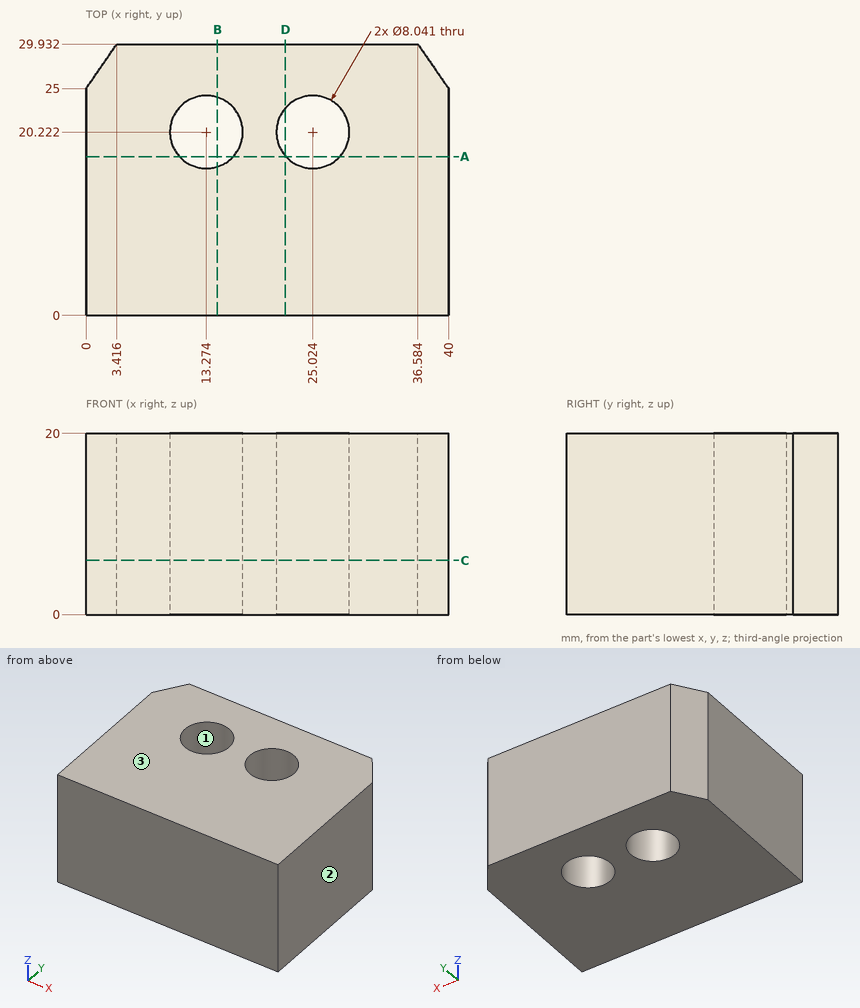
Study the drawing (mm; zero at the part's minimum x, y, z) and answer. Coordinates: 2 decimals unless noted, no trailing zeros. Write each loop counter-clockwise with the first axis right and the second up, starting at its lowest first coordinate (ties: lowest second). Pieces come first, ordered by that corner, then holes.
Q1. The mould has two halves that part along X. Classify the marked faces 1, 2 and 3: released by +X, released by -X, zero draft, split by the parting line, or undercut.
Returned:
face 1: undercut
face 2: released by +X
face 3: zero draft
Q2. Section B-B, the plane x = 14.5 is taken. Write down the section's boundary in (y, z).
Returned:
outline: (0, 0) - (16.39, 0) - (16.39, 20) - (0, 20) - close; (24.05, 0) - (29.93, 0) - (29.93, 20) - (24.05, 20) - close
Q3. Find the intervals of material crossed by line 1 along X through (y, z) = (22, 16.25); line 2 along X through (y, z) = (21, 2.25); line 3 along Y through (x, z) = (25, 11.5), in increasing order.
Returned:
line 1: x = 0 to 9.67, 16.88 to 21.42, 28.63 to 40
line 2: x = 0 to 9.33, 17.22 to 21.08, 28.97 to 40
line 3: y = 0 to 16.2, 24.24 to 29.93
Q4. Section C-C, the plane z = 6 is taken. Write down the section's boundary in (x, y) (1 decimal).
Returned:
outline: (0, 0) - (40, 0) - (40, 25) - (36.6, 29.9) - (3.4, 29.9) - (0, 25) - close; hole circle Ø8 at (13.3, 20.2); hole circle Ø8 at (25, 20.2)
Q5. Section D-D, the plane x = 22 is taken. Write down the section's boundary in (y, z).
Returned:
outline: (0, 0) - (17.57, 0) - (17.57, 20) - (0, 20) - close; (22.87, 0) - (29.93, 0) - (29.93, 20) - (22.87, 20) - close
Q6. Section A-A, the plane y = 17.5 is taken. Write down the section's boundary in (x, z) (1 decimal).
Returned:
outline: (0, 0) - (10.3, 0) - (10.3, 20) - (0, 20) - close; (16.2, 0) - (22.1, 0) - (22.1, 20) - (16.2, 20) - close; (28, 0) - (40, 0) - (40, 20) - (28, 20) - close
